Geometry check sheet. Reference: the model listing, model coordinates, mm. A direction names the side the tool comes from. Coordinates: 2 decimals unless noted, no trailing zeros. Write each loop counter-clockwise with the first axis right and the second up, starting at its lowest first coordinate (ties: lowest second). Pieces come first, ordered by that corner, then holes. Notation, with made-up numbers: (-24, 70) -> (31, 70) arc R29 cw to (31, 97) -> close; hole circle Ø5 at (68.25, 80). An arc over 180 degrees is marked (long way). Answer in a Markdown table with one row per item. Add a question column.
Q1. Section check C-C, the plane x = -10.5. Record the boundary of the cut face in (y, z).
Q2. Gauge pin test, flat ends, axial feed: P1, Ø2, axis at y = -64, z = 878, coming from the +X side; P2, Ø3, axis at x = -398, y = 1.5, coming from the -Z side; P3, Ø12, axis at x = 293, y = 203.5, coming from the -Z side. Record the tip position at first contact, or that the pin passes through.
Q3. Section check A-A, the plane z = 638.5. Record the boundary of the cut face in (x, y).
Q4. Tool access check on faces 1 (the face through (-998, -7, 380)), 2 (the face through (-786.129, 7, 1274.467)). Record the directions out of +Z, -Z, +X, -X, +Y, -Y that give a thin tool (end or side, any length) a straight path to the whole face; none if there is none.
Q5. Thickness scan on line 1 (X direction, y = 5.5, z = 756.5); line 2 (X direction, y = 427.5, z = 696); line 3 (Z direction, x = -267.5, y = -459). Record the ranges inside material, lowest first.
Q6. Release check for a two-part mould opening along X. For faces 3 (the face through (-4, -7, 1500)), 4 (the face through (1000, -7, 370)), 5 (the face through (784.7, -7, 1273.07)) record: pulls with the +X half, pulls with the -X half, needs draft (parallel to the pull), parting line crosses it, or undercut.
Q7. Section check B-B, the plane y = -135. Record the boundary of the cut face in (x, z).
```python
from build123d import *

# Parameters (mm, degrees)
F0_W     = 2000
F0_H     = 1500
F1_DEPTH = 500
F2_R     = 750
F4_DEPTH = 1000.001


# Not quite as in the source:
# - a feature names something its author has since deleted; it is built from what else it names


with BuildPart() as f1:
    # F0 (on Front) → F1 (new body, symmetric)
    with BuildSketch(Plane.XZ):
        with Locations((0, 750)):
            Rectangle(F0_W, F0_H)
    extrude(amount=F1_DEPTH, both=True)

    # F2
    f2_edges = [f1.edges().sort_by_distance(p)[0] for p in [
        (-1000, 0, 1500),
        (1000, 0, 1500),
    ]]
    fillet(f2_edges, radius=F2_R)

    # F3 (on face) → F4 (cut, through all)
    with BuildSketch(Plane.XZ.offset(500)):
        with BuildLine():
            ThreePointArc((-250, 1498), (-778.9158723275, 1278.9158723275), (-998, 750))
            Line((-998, 750), (-998, -0.5737363658))
            Line((-998, -0.5737363658), (998, -0.5742163858))
            Line((998, -0.5742163858), (998, 750))
            ThreePointArc((998, 750), (778.9158723275, 1278.9158723275), (250, 1498))
            Line((250, 1498), (-250, 1498))
        make_face()
    extrude(amount=-F4_DEPTH, mode=Mode.SUBTRACT)


solid = f1.part
```
Calculated:
| question | item | result |
|---|---|---|
| 1 | outline | (-500, 1498) -> (500, 1498) -> (500, 1500) -> (-500, 1500) -> close |
| 2 | P1 | stops at x = 989.17 |
| 2 | P2 | stops at z = 1482.91 |
| 2 | P3 | stops at z = 1496.39 |
| 3 | outline | (-1000, -500) -> (-998, -500) -> (-998, 500) -> (-1000, 500) -> close; (998, -500) -> (1000, -500) -> (1000, 500) -> (998, 500) -> close |
| 4 | face 1 | -Z, +Y, -Y |
| 4 | face 2 | +Z, -X, +Y, -Y |
| 5 | line 1 | x = -999.97 to -997.97, 997.97 to 999.97 |
| 5 | line 2 | x = -1000 to -998, 998 to 1000 |
| 5 | line 3 | z = 1497.8 to 1499.8 |
| 6 | face 3 | needs draft |
| 6 | face 4 | pulls with the +X half |
| 6 | face 5 | undercut |
| 7 | outline | (-1000, 0) -> (-998, 0) -> (-998, 750) arc R748 cw to (-250, 1498) -> (250, 1498) arc R748 cw to (998, 750) -> (998, 0) -> (1000, 0) -> (1000, 750) arc R750 ccw to (250, 1500) -> (-250, 1500) arc R750 ccw to (-1000, 750) -> close |
